Geometry check sheet. Reference: the model listing, model coordinates, mm. A direction names the side the tool comes from. Coordinates: 2 decimals unless noted, no trailing zeros. Write each loop counter-clockwise with the first axis right and the second up, starting at its lowest first coordinate (ties: lowest second). Pieces come first, ordered by that corner, then holes. Notation, with made-up numbers: M 5,82.25 L 30,82.25 A8 ccw 30,88.25 Z; hole C 18.25,1.5 d6. An arc over 180 degrees is marked long. Write item = value, one per line. Start each with the question number.
```python
from build123d import *

# Parameters (mm, degrees)
F1_DEPTH = 63.5
F0_W     = 25.4
F0_H     = 19.05
F2_DEPTH = 25.4
F3_DEPTH = 7.9375
F4_R     = 5.08


with BuildPart() as f1:
    # F0 (on Front) → F1 (new body, symmetric)
    with BuildSketch(Plane.XZ):
        Polygon((-41.275, -9.525), (41.275, -9.525), (41.275, 9.525), (22.225, 9.525), (-41.275, 9.525), align=None)
    extrude(amount=F1_DEPTH, both=True)

    # F0 (on Front) → F2 (join, symmetric)
    with BuildSketch(Plane.XZ):
        with BuildLine():
            Line((22.225, 9.525), (41.275, 9.525))
            Line((41.275, 9.525), (41.275, 27.0002))
            ThreePointArc((41.275, 27.0002), (45.9246798487, 38.2255201513), (57.15, 42.8752))
            Line((57.15, 42.8752), (60.325, 42.8752))
            Line((60.325, 42.8752), (60.325, 61.9252))
            Line((60.325, 61.9252), (57.15, 61.9252))
            ThreePointArc((57.15, 61.9252), (32.4542956671, 51.6959043329), (22.225, 27.0002))
            Line((22.225, 27.0002), (22.225, 9.525))
        make_face()
        with Locations((73.025, 52.4002)):
            Rectangle(F0_W, F0_H)
    extrude(amount=F2_DEPTH, both=True)

    # F0 (on Front) → F3 (join, symmetric)
    with BuildSketch(Plane.XZ):
        with BuildLine():
            add(Edge.make_bspline(
                [(-41.275, 9.525), (-33.7711833417, 32.2572402656), (0, 65.9977197647), (57.15, 61.9252)],
                knots=[0, 0, 0, 0, 111.5045361635, 111.5045361635, 111.5045361635, 111.5045361635], degree=3))
            Line((-41.275, 9.525), (22.225, 9.525))
            Line((22.225, 9.525), (22.225, 27.0002))
            ThreePointArc((22.225, 27.0002), (32.4542956671, 51.6959043329), (57.15, 61.9252))
        make_face()
    extrude(amount=F3_DEPTH, both=True)

    # F4
    f4_edges = [f1.edges().sort_by_distance(p)[0] for p in [
        (41.275, -63.5, 0),
        (41.275, 63.5, 0),
        (-41.275, 63.5, 0),
        (-41.275, -63.5, 0),
    ]]
    fillet(f4_edges, radius=F4_R)


solid = f1.part
```
Q1. Scan lines: L1, parallel to Z at x = 18, y = 57 (3 decimals); L2, parallel to Y at x = -28, z = 15; L3, parallel to Y at x = 33.5, z = 27. Record each from-to range of solid material in increasing order.
Q2. Cross-section at C-C on y = 32.5. Enter the section's corners in (x, z) (3 decimals).
Q3. Cross-section at A-A on y = 13. Enter the section's corners in (x, z) (3 decimals), and give its area (3 significant figures).
Q4. Gauge pin test, flat ends, axial feed: pin 1 (11 mm diameter, centred on y = 26, z = 5.5, fed in from +X) (3 decimals); pin 2 (6 mm diameter, centred on x = 39, y = -28, fed in from +Z); pin 3 (19 mm diameter, centred on y = 18, z = 20.5, fed in from -X) (3 decimals). Record the tip position at first contact, or that the pin passes through.
Q5. Set-up check for faces 1 (the face through (-2, 7.938, 32)), 2 (the face through (41.275, -1, 4)), 3 (the face through (32.73, -16.79, 51.97)), 4 (the face through (46, 25.4, 42)), 5 (the face through (46, -25.4, 42)): record each of +Z, -Z, +X, -X, +Y, -Y from which the full face is reachable in a straight line by a thin tool's end or side.
Q6. Cross-section at B-B on x = 60. Enter the section's corners in (y, z).
Values found:
q1.L1 = -9.525 to 9.525
q1.L2 = -7.94 to 7.94
q1.L3 = -25.4 to 25.4
q2.outline = M -41.275,-9.525 L 41.275,-9.525 L 41.275,9.525 L -41.275,9.525 Z
q3.outline = M -41.275,-9.525 L 41.275,-9.525 L 41.275,27 A15.875 cw 57.15,42.875 L 85.725,42.875 L 85.725,61.925 L 57.15,61.925 A34.925 ccw 22.225,27 L 22.225,9.525 L -41.275,9.525 Z
q3.area = 3,210 mm²
q4.pin_1 = 41.275
q4.pin_2 = 57.7
q4.pin_3 = 22.225
q5.face_1 = +Z, -X, +Y
q5.face_2 = -Z, +X, +Y, -Y
q5.face_3 = +Z, -X, -Y
q5.face_4 = +Z, +X, -X, +Y
q5.face_5 = +Z, +X, -X, -Y
q6.outline = M -25.4,42.88 L 25.4,42.88 L 25.4,61.93 L -25.4,61.93 Z
